Can you work these out from the model? Positions are in its coordinate system, mm. Round coordinates to 2 decimals unless told otherwise and drop trailing zeros. Order: outer loops, then holes, each group sorted by start corner. A loop starts at its lowest first (then second) coordinate and runs counter-clockwise, first axis right, second up.
Q1. If we section it at B-B (x = 0.65): Count the separate pieces of the cut face and the enclosed holes in it, plus the area to 3 significant figures.
Q2. We'd pull the mould along Z, two halves only. Please class faces 1 (the face through (1, 1, 0)), 2 (the face through (-0.01, -79.81, -13.44)), 3 (the face through (0.014, 81.787, 10.202)): pulls with the +Z half, pulls with the -Z half, needs draft (parallel to the pull), parting line crosses it, or undercut.
Q3. If we section it at C-C (z = 13): Please give me the cut outline in (x, y), plus the area to 3 significant figures.
Q4. If we section it at A-A (y = -73.75): Please give me the cut outline in (x, z) (3 decimals), plus the area to 3 significant figures.
Q5. If I drill on line 1 (Z direction, x = -0.6, y = -73.75) (3 decimals); line 2 (Y direction, x = 0.1, z = 9.5); line 3 (Y direction, x = -0.3, z = -10), over which ranges is the centre line in solid material (lowest first)?
Q6. Will this pin go through, and if not, where does the flat tip stop? P1, Ø0.6, axis at x = -0.5, z = 0.5, coming from the -Y side.
from build123d import *

# Parameters (mm, degrees)
SKETCH_1_W          = 35
SKETCH_1_H          = 167.5
EXTRUDE_1_DEPTH     = 1
SKETCH_2_W          = 2.45
SKETCH_2_H          = 5
CUT_EXTRUDE_1_DEPTH = 3
SKETCH_3_R          = 0.6
CUT_EXTRUDE_2_DEPTH = 3
SKETCH_5_W          = 2.45
SKETCH_5_H          = 5
CUT_EXTRUDE_4_DEPTH = 3
SKETCH_6_R          = 0.6
CUT_EXTRUDE_5_DEPTH = 3
SKETCH_7_R          = 1.55
CUT_EXTRUDE_6_DEPTH = 3
CHAMFER_1_SIZE      = 8
CUT_EXTRUDE_8_DEPTH = 3
FILLET_1_R          = 1
SKETCH_11_R         = 1.55
CUT_EXTRUDE_9_DEPTH = 3


with BuildPart() as part:
    # 草图1 → 凸台-拉伸1 (new body, symmetric)
    with BuildSketch(Plane(origin=(0, 0, 0), x_dir=(0, 0, -1), z_dir=(1, 0, 0))):
        Rectangle(SKETCH_1_W, SKETCH_1_H)
    extrude(amount=EXTRUDE_1_DEPTH, both=True)

    # 草图2 → 切除-拉伸1 (cut, through all)
    with BuildSketch(Plane(origin=(1, 0, 0), x_dir=(0, 0, -1), z_dir=(1, 0, 0))):
        with Locations((0, -81.25)):
            Rectangle(SKETCH_2_W, SKETCH_2_H)
    extrude(amount=-CUT_EXTRUDE_1_DEPTH, mode=Mode.SUBTRACT)

    # 草图3 → 切除-拉伸2 (cut, through all)
    with BuildSketch(Plane(origin=(1, 0, 0), x_dir=(0, 0, -1), z_dir=(1, 0, 0))):
        with Locations((-1.225, -79.35)):
            Circle(SKETCH_3_R)
        with Locations((1.225, -79.35)):
            Circle(SKETCH_3_R)
    extrude(amount=-CUT_EXTRUDE_2_DEPTH, mode=Mode.SUBTRACT)

    # 草图5 → 切除-拉伸4 (cut, through all)
    with BuildSketch(Plane(origin=(1, 0, 0), x_dir=(0, 0, -1), z_dir=(1, 0, 0))):
        with Locations((0, -66.2)):
            Rectangle(SKETCH_5_W, SKETCH_5_H)
    extrude(amount=-CUT_EXTRUDE_4_DEPTH, mode=Mode.SUBTRACT)

    # 草图6 → 切除-拉伸5 (cut, through all)
    with BuildSketch(Plane(origin=(1, 0, 0), x_dir=(0, 0, -1), z_dir=(1, 0, 0))):
        with Locations((-1.225, -64.3)):
            Circle(SKETCH_6_R)
        with Locations((-1.225, -68.1)):
            Circle(SKETCH_6_R)
        with Locations((1.225, -64.3)):
            Circle(SKETCH_6_R)
        with Locations((1.225, -68.1)):
            Circle(SKETCH_6_R)
    extrude(amount=-CUT_EXTRUDE_5_DEPTH, mode=Mode.SUBTRACT)

    # 草图7 → 切除-拉伸6 (cut, through all)
    with BuildSketch(Plane(origin=(1, 0, 0), x_dir=(0, 0, -1), z_dir=(1, 0, 0))):
        with Locations((-4.225, -73.75)):
            Circle(SKETCH_7_R)
        with Locations((4.225, -73.75)):
            Circle(SKETCH_7_R)
    extrude(amount=-CUT_EXTRUDE_6_DEPTH, mode=Mode.SUBTRACT)

    # 倒角1
    chamfer_1_edges = [part.edges().sort_by_distance(p)[0] for p in [
        (0, -83.75, -17.5),
        (0, -83.75, 17.5),
    ]]
    chamfer(chamfer_1_edges, length=CHAMFER_1_SIZE)

    # 草图10 → 切除-拉伸8 (cut, through all)
    with BuildSketch(Plane(origin=(1, 0, 0), x_dir=(0, 0, -1), z_dir=(1, 0, 0))):
        Polygon((7.5, 83.75), (-7.5, 83.75), (-5, 73.75), (5, 73.75), align=None)
    extrude(amount=-CUT_EXTRUDE_8_DEPTH, mode=Mode.SUBTRACT)

    # 圆角1
    fillet_1_edges = [part.edges().sort_by_distance(p)[0] for p in [
        (0, 73.75, 5),
        (0, 73.75, -5),
    ]]
    fillet(fillet_1_edges, radius=FILLET_1_R)

    # 草图11 → 切除-拉伸9 (cut, through all)
    with BuildSketch(Plane(origin=(1, 0, 0), x_dir=(0, 0, -1), z_dir=(1, 0, 0))):
        with Locations((-10, 80.25)):
            Circle(SKETCH_11_R)
        with Locations((10, 80.25)):
            Circle(SKETCH_11_R)
    extrude(amount=-CUT_EXTRUDE_9_DEPTH, mode=Mode.SUBTRACT)


solid = part.part
Solution:
1. separate pieces: 1
1. enclosed holes: 5
1. area: 5,620 mm2
2. face 1: needs draft
2. face 2: pulls with the -Z half
2. face 3: undercut
3. outline: (-1, -80.25) - (1, -80.25) - (1, 83.75) - (-1, 83.75) - close
3. area: 328 mm2
4. outline: (-1, -17.5) - (1, -17.5) - (1, -5.775) - (-1, -5.775) - close; (-1, -2.675) - (1, -2.675) - (1, 2.675) - (-1, 2.675) - close; (-1, 5.775) - (1, 5.775) - (1, 17.5) - (-1, 17.5) - close
4. area: 57.6 mm2
5. line 1: z = -17.5 to -5.775, -2.675 to 2.675, 5.775 to 17.5
5. line 2: y = -83.75 to 78.78, 81.72 to 83.75
5. line 3: y = -83.25 to 78.7, 81.8 to 83.75
6. P1: stops at y = -78.75
